from build123d import *

# Parameters (mm, degrees)
F0_R          = 43.688
F2_DEPTH      = 76.1238
F2_DEPTH_BACK = 76.1238
F1_R          = 43.688
F3_DEPTH      = 54.356
F4_R          = 50.8
F4_R_2        = 43.688
F5_DEPTH      = 50.8


with BuildPart() as f2:
    # F0 (on Front) → F2 (new body, two sides)
    with BuildSketch(Plane.XZ) as f2_sk:
        Circle(F0_R)
    extrude(amount=F2_DEPTH)
    extrude(f2_sk.sketch, amount=-F2_DEPTH_BACK)

    # F1 (on Top) → F3 (join)
    with BuildSketch(Plane.XY):
        Circle(F1_R)
    extrude(amount=F3_DEPTH)

    # F4 (on face) → F5 (join)
    with BuildSketch(Plane.XY.offset(54.356)):
        Circle(F4_R)
        Circle(F4_R_2, mode=Mode.SUBTRACT)
        Circle(F4_R_2)
    extrude(amount=F5_DEPTH)


solid = f2.part
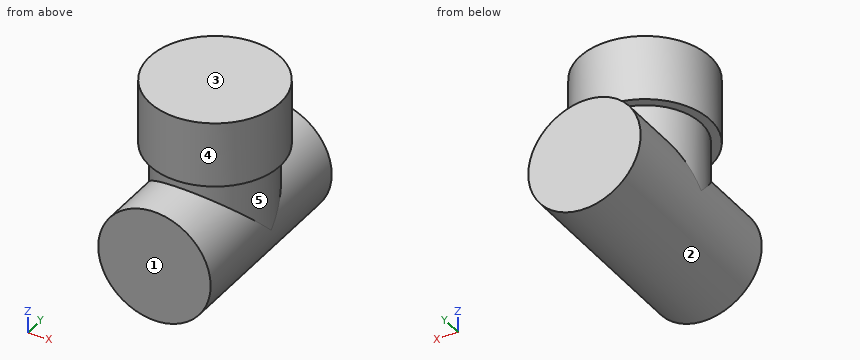
The model under review builds one solid part; all positions refer to its coordinate system, in mm. Face numbers are marked on the shaded views. A direction names the side the tool comes from. Give positions to 0.01 mm unless a question says otherwise; leave off trailing zeros. Loops run counter-clockwise (first coordinate to the right, second up) from the corner with the lowest first, then second, coordinate; pieces in that order, holes last. Notation, with made-up numbers: (-3, 41.25) -> (11, 41.25) arc R8 cw to (11, 51.25) -> close; hole circle Ø7 at (-6, 9.25). An arc over 180 degrees is marked (long way). Put each result on its own line as item: value. Start each with the question number.
1. We need section C-C on z = 6.5. State the section outline as (x, y) points, then the cut area to 3 significant figures.
2. For the marked faces 1 and 2, list the 3-axis set-ups (+Z, -Z, +X, -X, +Y, -Y) from which the entire face can be reached by the end or side of a thin tool; tool diameter is ignored.
3. Wall thickness on probe 1 along Z at (x, y) = (0.5, 21.5); probe 2 along Z at (x, y) = (-25, 38); probe 3 along Z at (x, y) = (-44, -20.5): over which ranges is each line inside the solid? List them lowest first.
4. We need section A-A on y = 0. State the section outline as (x, z) points.
5. Clearance check with flat-ended pins moving along their axes: P1, Ø1, axis at x = 1, y = 2, coming from the -Z side; P2, Ø3, axis at y = 57, z = 10.5, coming from the -X side; P3, Ø8, axis at y = -12, z = 66.5, coming from the -X side. State where each tip first meets the part, or that it passes through.
6. We need section B-B on x = 0. State the section outline as (y, z) points, then the cut area to 3 significant figures.
7. We need section D-D on x = 25. State the section outline as (y, z) points.
8. Mouldability with a two-part tool opening along Z and no side actions: class the marked faces 3, 4 and 5 as released by +Z, released by -Z, zero draft, split by the parting line, or undercut.
Determined:
1. outline: (-43.2, -76.12) -> (43.2, -76.12) -> (43.2, -6.5) arc R43.69 ccw to (43.2, 6.5) -> (43.2, 76.12) -> (-43.2, 76.12) -> (-43.2, 6.5) arc R43.69 ccw to (-43.2, -6.5) -> close
1. area: 13,200 mm^2
2. face 1: +Z, -Z, +X, -X, -Y
2. face 2: none
3. probe 1: -43.69 to 105.16
3. probe 2: -35.83 to 35.83, 54.36 to 105.16
3. probe 3: 54.36 to 105.16
4. outline: (-50.8, 54.36) -> (-43.69, 54.36) -> (-43.69, 0) arc R43.69 ccw to (43.69, 0) -> (43.69, 54.36) -> (50.8, 54.36) -> (50.8, 105.16) -> (-50.8, 105.16) -> close
5. P1: z = -43.69
5. P2: x = -42.75
5. P3: x = -50.17
6. outline: (-76.12, -43.69) -> (76.12, -43.69) -> (76.12, 43.69) -> (43.69, 43.69) -> (43.69, 54.36) -> (50.8, 54.36) -> (50.8, 105.16) -> (-50.8, 105.16) -> (-50.8, 54.36) -> (-43.69, 54.36) -> (-43.69, 43.69) -> (-76.12, 43.69) -> close
6. area: 19,400 mm^2
7. outline: (-76.12, -35.83) -> (76.12, -35.83) -> (76.12, 35.83) -> (35.83, 35.83) -> (35.83, 54.36) -> (44.22, 54.36) -> (44.22, 105.16) -> (-44.22, 105.16) -> (-44.22, 54.36) -> (-35.83, 54.36) -> (-35.83, 35.83) -> (-76.12, 35.83) -> close
8. face 3: released by +Z
8. face 4: zero draft
8. face 5: undercut
